Geometry: final body of the model. Coordinates: model frame, mm. A direction names the side the tool comes from. Coordinates: 2 decimals unless noted, no trailing zeros. Write each loop counter-clockwise with the first axis right and the second up, starting at its lowest first coordinate (ties: lowest second). Pieces come first, ordered by that corner, then holes. Notation, with made-up numbers: (-24.5, 82) -> (-8.5, 82) arc R15 ccw to (-8.5, 105) -> close; hole circle Ø1 at (-22, -30.75). An arc over 180 degrees is marked (long way). One line per item, written item: value. Start each with the question number.
from build123d import *

# Parameters (mm, degrees)
F0_R     = 27.361448
F0_R_2   = 20
F1_DEPTH = 5
F2_W     = 3.56566
F2_H     = 20
F3_DEPTH = 30
F4_R     = 4
F5_DEPTH = 25
F6_R     = 8


with BuildPart() as f1:
    # F0 (on Top) → F1 (new body)
    with BuildSketch(Plane.XY):
        Circle(F0_R)
        Circle(F0_R_2, mode=Mode.SUBTRACT)
    extrude(amount=F1_DEPTH)

    # F2 (on face) → F3 (join)
    with BuildSketch(Plane(origin=(0, 0, 0), x_dir=(1, 0, 0), z_dir=(0, 0, -1))):
        with Locations((-23.004174, 0)):
            Rectangle(F2_W, F2_H)
    extrude(amount=F3_DEPTH)

    # F4 (on face) → F5 (cut)
    with BuildSketch(Plane(origin=(-24.787004, 0, 0), x_dir=(0, -1, 0), z_dir=(-1, 0, 0))):
        with Locations((0, -20)):
            Circle(F4_R)
    extrude(amount=-F5_DEPTH, mode=Mode.SUBTRACT)

    # F6
    f6_edges = [f1.edges().sort_by_distance(p)[0] for p in [
        (-23.004174, -10, -30),
        (-23.004174, 10, -30),
    ]]
    fillet(f6_edges, radius=F6_R)


solid = f1.part
Q1. Line query: L1, parallel to Y at x = 0, z = 2.3; L2, parallel to Z at x = 9.5, y = -23.5; L3, parallel to X at y = -0.5, z = -4.5. Output: solid intervals per line, ascending. Write a range as from..to.
Q2. First-contact query: P1, Ø16, axis at y = 0, z = -13, coming from the +X side; P2, Ø16, axis at y = -3.5, z = -20, coming from the -X side; P3, Ø3, axis at x = -23.5, z = -12, coming from the +Y side. Flat tips, straight axial feed; report the tip coordinate or a pass-through.
Q3. Access query for faces 1 (the flat face through (-24.787, 0, -15)), 2 (the flat face through (-21.221, 0, -15)), 3 (the flat face through (-23, 10, -11)), 4 (the cylindrical face through (26.098, 8.219, 2.465)), 5 (the flat face through (-23, -10, -11)). Directions: +Z, -Z, +X, -X, +Y, -Y. A direction counts if a zero-diameter tool reaches every point of the face in a straight line with its end or side. Return the directions, or none.
Q4. Cut plane C-C on x = 0. Output: boundary loops of the cut face in (y, z), and give its area (3 significant figures).
Q5. Draft query along Y for faces 6 (the cylindrical face through (-22.979, 7.719, -27.594)), 7 (the cylindrical face through (-22.979, -7.719, -27.594)), 8 (the cylindrical face through (-4.336, -19.524, 2.465)). Return one class per face: pulls with the +Y half, pulls with the -Y half, needs draft (parallel to the pull), parting line crosses it, or undercut.
Q6. Cut plane D-D on y = 7. Output: boundary loops of the cut face in (x, z) (3 decimals).
Q7. Cut plane A-A on y = 0. Output: boundary loops of the cut face in (x, z), and give its area (3 significant figures).
Q8. Cut plane B-B on z = -20. Output: boundary loops of the cut face in (x, y), and give its area (3 significant figures).
Solution:
1. L1: -27.36..-20, 20..27.36
1. L2: 0..5
1. L3: -24.79..-21.22
2. P1: x = -21.22
2. P2: x = -24.79
2. P3: y = 10
3. face 1: -Z, -X, +Y, -Y
3. face 2: -Z, +X, +Y, -Y
3. face 3: -Z, +X, -X, +Y
3. face 4: +Z, -Z
3. face 5: -Z, +X, -X, -Y
4. outline: (-27.36, 0) -> (-20, 0) -> (-20, 5) -> (-27.36, 5) -> close; (20, 0) -> (27.36, 0) -> (27.36, 5) -> (20, 5) -> close
4. area: 73.6 mm²
5. face 6: pulls with the +Y half
5. face 7: pulls with the -Y half
5. face 8: undercut
6. outline: (-26.451, 0) -> (-24.787, 0) -> (-24.787, -28.245) -> (-21.221, -28.245) -> (-21.221, 0) -> (-18.735, 0) -> (-18.735, 5) -> (-26.451, 5) -> close; (18.735, 0) -> (26.451, 0) -> (26.451, 5) -> (18.735, 5) -> close
7. outline: (-27.36, 0) -> (-24.79, 0) -> (-24.79, -16) -> (-21.22, -16) -> (-21.22, 0) -> (-20, 0) -> (-20, 5) -> (-27.36, 5) -> close; (-24.79, -30) -> (-21.22, -30) -> (-21.22, -24) -> (-24.79, -24) -> close; (20, 0) -> (27.36, 0) -> (27.36, 5) -> (20, 5) -> close
7. area: 152 mm²
8. outline: (-24.79, -10) -> (-21.22, -10) -> (-21.22, -4) -> (-24.79, -4) -> close; (-24.79, 4) -> (-21.22, 4) -> (-21.22, 10) -> (-24.79, 10) -> close
8. area: 42.8 mm²
